Model file for the job. Use its own axes, mm. A direction names the side the tool comes from. Give positions to 0.01 mm unless a question says otherwise; leave off trailing zeros. Write each loop counter-clockwise with the first axis right and the second up, starting at its lowest first coordinate (ties: lowest second). Pieces come first, ordered by that corner, then holes. Notation, with made-up numbers: (12, -10) - (68, -10) arc R18 ccw to (68, 2) - close; hole circle Ø1 at (12, -37). An arc over 180 degrees is marked (long way). One line per item, written item: value. Start each with the question number.
(1) Cut at B-B, the plane x = 104.5. List the corners of the cut face in (y, z).
(2) 3-axis set-ups, long thin cutter, end or side, ignore diameter. For faces 1 (the face through (40, -1148, 115.5)), 2 (the face through (37, -1148, 120)), 3 (the face through (70, 0, 132)): which of +Z, -Z, +X, -X, +Y, -Y reach the whole face in a straight line?
(3) Probe L1, parallel to X at y = -608, z = 137; L2, parallel to X at y = -1841, z = 122.5; L3, parallel to Z at x = 85.5, y = -1626. List the from-to ranges inside material, lowest first.
(4) Cut at A-A, the plane y = -1002. List the corners of the cut face in (x, z).
(5) Mould opens along X. For faces 4 (the face through (108, -1148, 151.75)), 5 (the face through (107, -1148, 147.25)) say: pulls with the +X half, pulls with the -X half, needs draft (parallel to the pull), parting line crosses it, or undercut.
(6) Drop flat-ended pins along their axis: P1, Ø1.3, axis at x = 145.5, y = -1695, coming from the -Z side; P2, Ø24, axis at y = -641.5, z = 135, coming from the -X side; P3, Ø3, axis at x = 19.5, z = 113, coming from the -Y side; P4, Ø12.5, axis at y = -1164.5, z = 103.5, coming from the +X side. Give the stop position or say it passes through.
from build123d import *

# Parameters (mm, degrees)
F1_DEPTH = 2329


with BuildPart() as f1:
    # F0 (on Front) → F1 (new body)
    with BuildSketch(Plane.XZ):
        with BuildLine():
            Line((147.5, 120), (147.5, 146.75))
            ThreePointArc((147.5, 146.75), (146.035534, 150.285534), (142.5, 151.75))
            Line((142.5, 151.75), (73, 151.75))
            ThreePointArc((73, 151.75), (69.464466, 150.285534), (68, 146.75))
            Line((68, 146.75), (68, 125))
            ThreePointArc((68, 125), (66.535534, 121.464466), (63, 120))
            Line((63, 120), (9.5, 120))
            ThreePointArc((9.5, 120), (5.964466, 118.535534), (4.5, 115))
            Line((4.5, 115), (4.5, 94.6))
            Line((4.5, 94.6), (9, 94.6))
            Line((9, 94.6), (9, 110.5))
            ThreePointArc((9, 110.5), (10.464466, 114.035534), (14, 115.5))
            Line((14, 115.5), (67.5, 115.5))
            ThreePointArc((67.5, 115.5), (71.035534, 116.964466), (72.5, 120.5))
            Line((72.5, 120.5), (72.5, 142.25))
            ThreePointArc((72.5, 142.25), (73.964466, 145.785534), (77.5, 147.25))
            Line((77.5, 147.25), (138, 147.25))
            ThreePointArc((138, 147.25), (141.535534, 145.785534), (143, 142.25))
            Line((143, 142.25), (143, 120))
            Line((143, 120), (147.5, 120))
        make_face()
    extrude(amount=F1_DEPTH)


solid = f1.part
Answers follow:
1. outline: (-2329, 147.25) - (0, 147.25) - (0, 151.75) - (-2329, 151.75) - close
2. face 1: -Z, +X, +Y, -Y
2. face 2: +Z, -X, +Y, -Y
2. face 3: +Z, -Z, +X, -X, +Y
3. L1: x = 68 to 72.5, 143 to 147.5
3. L2: x = 67.33 to 72.5, 143 to 147.5
3. L3: z = 147.25 to 151.75
4. outline: (4.5, 94.6) - (9, 94.6) - (9, 110.5) arc R5 cw to (14, 115.5) - (67.5, 115.5) arc R5 ccw to (72.5, 120.5) - (72.5, 142.25) arc R5 cw to (77.5, 147.25) - (138, 147.25) arc R5 cw to (143, 142.25) - (143, 120) - (147.5, 120) - (147.5, 146.75) arc R5 ccw to (142.5, 151.75) - (73, 151.75) arc R5 ccw to (68, 146.75) - (68, 125) arc R5 cw to (63, 120) - (9.5, 120) arc R5 ccw to (4.5, 115) - close
5. face 4: needs draft
5. face 5: undercut
6. P1: stops at z = 120
6. P2: stops at x = 67.58
6. P3: passes through
6. P4: stops at x = 9
